Here's the drawing with two shaded views (mm, measured from the low corner). I have some questions. Give positions to 0.01 mm unless a question says otherwise; leave off trailing zeros. Write each loop counter-clockwise with the first axis right and the second up, starting at its lowest first coordinate (ties: lowest second). Pieces come first, ordered by that corner, then holes.
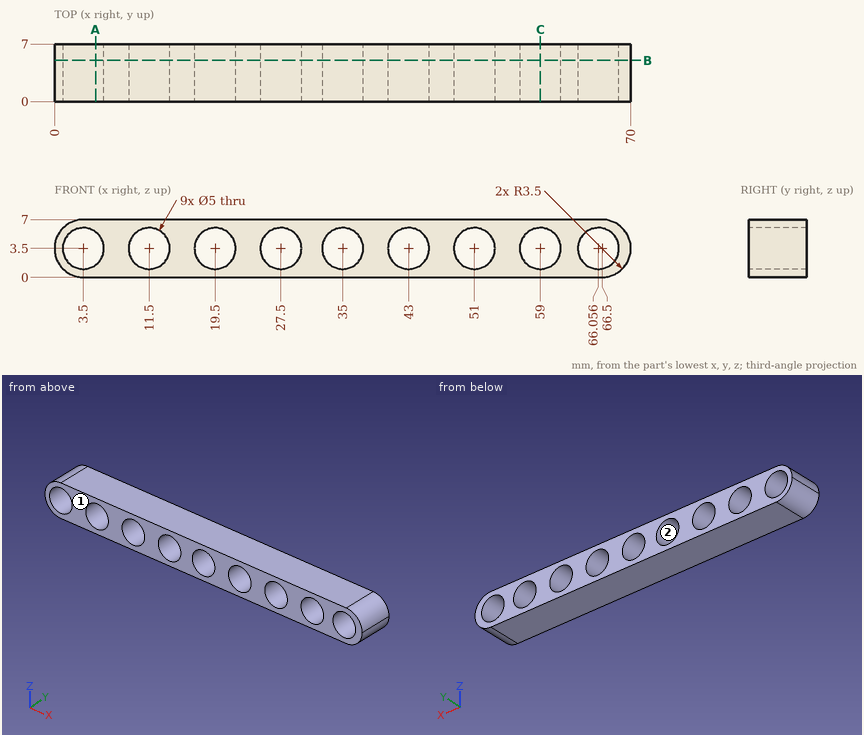
1) Please list where these lines run through material, in increasing order: L1, parallel to Z at x = 19.5, y = 4.25; L2, parallel to Z at x = 45, y = 3.5.
Values follow:
L1: z = 0 to 1, 6 to 7
L2: z = 0 to 2, 5 to 7
2) Suppose I cut it at A-A on x = 5. Write out the boundary of the cut face in (y, z).
Values follow:
outline: (0, 0) - (7, 0) - (7, 1.5) - (0, 1.5) - close; (0, 5.5) - (7, 5.5) - (7, 7) - (0, 7) - close
3) Suppose I cut it at C-C on x = 59. Write out the boundary of the cut face in (y, z), plus the area to 3 significant figures.
Values follow:
outline: (0, 0) - (7, 0) - (7, 1) - (0, 1) - close; (0, 6) - (7, 6) - (7, 7) - (0, 7) - close
area: 14.0 mm2
4) If we mould it in two halves opening along X, with no side actions, what happens to the marked faces 1 and 2? For each: +X half, -X half, draft (parallel to the pull), parting line (faces both ways), or undercut.
Values follow:
face 1: draft
face 2: undercut
5) Suppose I cut it at B-B on y = 5. State how many separate pieces and enclosed holes the cut face has, plus the area to 3 significant figures.
Values follow:
separate pieces: 1
enclosed holes: 9
area: 303 mm2
